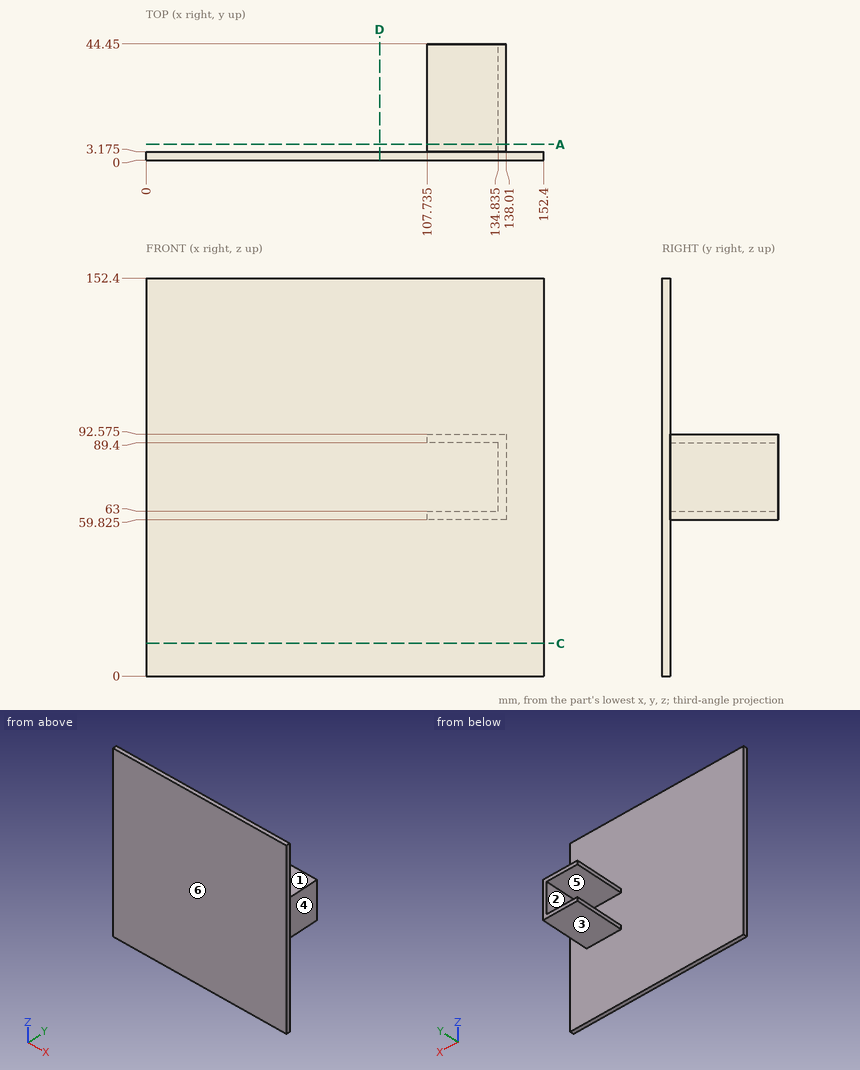
Could you check a few things on this drawing? It's one solid part, dimensions in mm from its lowest x, y, z. A direction names the side the tool comes from. Round coordinates to 2 decimals unless told otherwise and drop trailing zeros. Write each loop counter-clockwise with the first axis right and the second up, starting at its lowest first coordinate (ties: lowest second). Pieces come first, ordered by that corner, then holes. Notation, with made-up numbers: (-9.75, 87.25) -> (-0.75, 87.25) arc R30 cw to (-0.75, 109.25) -> close; hole circle Ø10 at (72.25, 29). An arc over 180 degrees is marked (long way). Use one line per item in the form item = value. Start each with the question number.
Q1. Imagine slicing it at C-C (z = 12.5). Please give me the cut outline in (x, y) (1 decimal), then the cut area to 3 significant figures.
Q2. If I drill on probe 1 along Z at (x, y) = (123.5, 21.5) (1 decimal); probe 2 along Y at (x, z) = (49, 40.5) (1 decimal); probe 3 along X at (y, z) = (33, 92) (1 decimal), over which ranges is the centre line in solid material (lowest first)? Write a range as [from, to].
Q3. We'd pull the mould along Z, two halves only. Please class the marked faces 1, 2, 3 and 4: +Z half, -Z half, draft (parallel to the pull), parting line (faces both ways), or undercut.
Q4. Imagine slicing it at A-A (y = 6). Please give me the cut outline in (x, z) (1 decimal).
Q5. Which directions (+Z, -Z, +X, -X, +Y, -Y) give clear straight access to the entire face, cutting with the end or side of a thin tool? Please do the marked faces 5 and 6.
Q6. Imagine slicing it at D-D (x = 89.5). Please give me the cut outline in (y, z) (1 decimal), then the cut area to 3 significant figures.
Q7. I'm going to push flat-ended pins straight in: P1, Ø15, axis at x = 128.5, y = 21.5, coming from the +Z side (1 decimal); P2, Ø1.5, axis at x = 102, z = 99.5, coming from the +Y side (1 decimal); P3, Ø2.5, axis at y = 31.5, z = 61, coming from the -X side (1 decimal). Where does each tip first touch, or does it pass through?
Worked out:
q1.outline = (0, 0) -> (152.4, 0) -> (152.4, 3.2) -> (0, 3.2) -> close
q1.area = 484 mm^2
q2.probe_1 = [59.8, 63], [89.4, 92.6]
q2.probe_2 = [0, 3.2]
q2.probe_3 = [107.7, 138]
q3.face_1 = +Z half
q3.face_2 = undercut
q3.face_3 = -Z half
q3.face_4 = draft
q4.outline = (107.7, 59.8) -> (138, 59.8) -> (138, 92.6) -> (107.7, 92.6) -> (107.7, 89.4) -> (134.8, 89.4) -> (134.8, 63) -> (107.7, 63) -> close
q5.face_5 = -X, +Y
q5.face_6 = +Z, -Z, +X, -X, -Y
q6.outline = (0, 0) -> (3.2, 0) -> (3.2, 152.4) -> (0, 152.4) -> close
q6.area = 484 mm^2
q7.P1 = 92.6
q7.P2 = 3.2
q7.P3 = 107.7
